Read the model definition and answer for the solid it produces. Units are mm, in the model's axes. Coordinates: 2 decimals unless noted, no trailing zeros. Loops run counter-clockwise (first coordinate to the right, second up) from the corner with the lowest first, then second, coordinate; pieces in that order, holes last. Notation, with made-up numbers: (-16, -14.5) -> (1, -14.5) arc R18 ccw to (1, 12.5) -> close; hole circle Ø3 at (70.25, 68). An arc over 180 degrees is marked (long way). Answer in a Markdown table with one row per item.
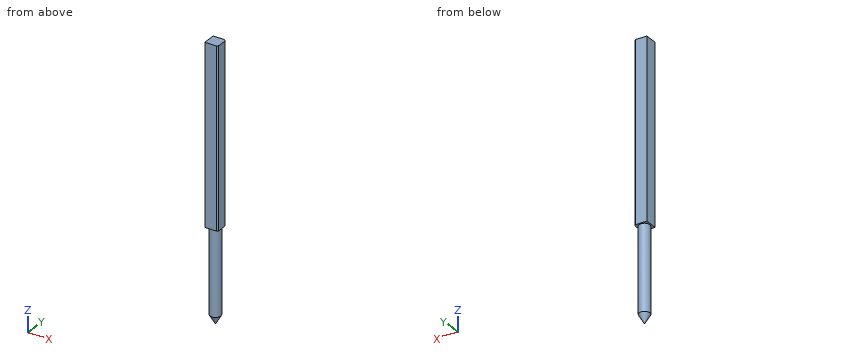
```python
from build123d import *

# Parameters (mm, degrees)
SKETCH1_W           = 6.1
SKETCH1_H           = 6.1
BOSS_EXTRUDE1_DEPTH = 84
SKETCH1_4_R         = 2.5
BOSS_EXTRUDE2_DEPTH = 40
CHAMFER_BASE_SIZE   = 0.686


with BuildPart() as part:
    # Sketch1 → Boss-Extrude1 (new body)
    with BuildSketch(Plane.XY):
        Rectangle(SKETCH1_W, SKETCH1_H)
    extrude(amount=BOSS_EXTRUDE1_DEPTH)

    # Sketch1<4> → Boss-Extrude2 (add)
    with BuildSketch(Plane.XY):
        Circle(SKETCH1_4_R)
    extrude(amount=-BOSS_EXTRUDE2_DEPTH)

    # Boss-Extrude3 cone 1 section (through the dimple's axis) → Boss-Extrude3 (revolve)
    with BuildSketch(Plane(origin=(0, 0, -40), x_dir=(0, -1, 0), z_dir=(1, 0, 0))):
        Polygon((0, 0), (2.5, 0), (0, 4.330127019), align=None)
    revolve(axis=Axis((0, 0, -40), (0, 0, -1)))

    # chamfer_base
    chamfer_base_edges = [part.edges().sort_by_distance(p)[0] for p in [
        (3.05, 3.05, 42),
        (3.05, -3.05, 42),
    ]]
    chamfer(chamfer_base_edges, length=CHAMFER_BASE_SIZE)


solid = part.part
```
1. Find the intervals of material crossed by probe 1 along Y at (x, z) = (0, -18); probe 2 along Z at (x, y) = (2.75, 0.5); probe 3 along X at (y, z) = (0.75, -25.5), in increasing order.
A:
| item | result |
|---|---|
| probe 1 | y = -2.5 to 2.5 |
| probe 2 | z = 0 to 84 |
| probe 3 | x = -2.38 to 2.38 |
2. Given pin 1 Ø3 at (x, y) = (0, -0.5) entering from -Z, flat-ended and moving along its own axis, determine where the tip first touches the part or whether it passes through.
A:
| item | result |
|---|---|
| pin 1 | stops at z = -44.33 |
3. A cutting plane is placed at A-A on z = -7. Give the vertices of the cut face in (x, y).
A:
| item | result |
|---|---|
| outline | circle Ø5 at (0, 0) |
